from build123d import *

# Parameters (mm, degrees)
SKETCH1_W                = 13
SKETCH1_H                = 35
SKETCH1_R                = 3.175
BOSS_EXTRUDE1_DEPTH      = 101.6
CUT_EXTRUDE1_DEPTH       = 9
M4_CLEARANCE_HOLE1_D     = 4.3
M4_CLEARANCE_HOLE1_DEPTH = 5
M4_CLEARANCE_HOLE1_TIP   = 1.291850331
M4_CLEARANCE_HOLE2_D     = 4.3
M4_CLEARANCE_HOLE2_DEPTH = 5
M4_CLEARANCE_HOLE2_TIP   = 1.291850331
FILLET1_R                = 3


with BuildPart() as part:
    # Sketch1 → Boss-Extrude1 (new body)
    with BuildSketch(Plane.XY):
        with Locations((6.5, 17.5)):
            Rectangle(SKETCH1_W, SKETCH1_H)
        with Locations((6.5, 30)):
            Circle(SKETCH1_R, mode=Mode.SUBTRACT)
    extrude(amount=BOSS_EXTRUDE1_DEPTH)

    # Sketch2 → Cut-Extrude1 (cut, symmetric)
    with BuildSketch(Plane.XY.offset(75.25)):
        Polygon((0, 30), (0, 35), (13, 35), (13, 30), (13, 23.5), (0, 23.5), align=None)
    extrude(amount=CUT_EXTRUDE1_DEPTH, both=True, mode=Mode.SUBTRACT)

    # M4 Clearance Hole1
    with Locations(Plane(origin=(0, 0, 0), x_dir=(-1, 0, 0), z_dir=(0, 0, -1))):
        with Locations((-6.579246302, 18), (-6.579246302, 6)):
            Hole(M4_CLEARANCE_HOLE1_D / 2, depth=M4_CLEARANCE_HOLE1_DEPTH)
            with Locations((0, 0, -(M4_CLEARANCE_HOLE1_DEPTH + M4_CLEARANCE_HOLE1_TIP / 2))):  # 118° drill point
                Cone(0, M4_CLEARANCE_HOLE1_D / 2, M4_CLEARANCE_HOLE1_TIP, mode=Mode.SUBTRACT)

    # M4 Clearance Hole2
    with Locations(Plane.XY.offset(101.6)):
        with Locations((6.579246302, 18), (6.579246302, 6)):
            Hole(M4_CLEARANCE_HOLE2_D / 2, depth=M4_CLEARANCE_HOLE2_DEPTH)
            with Locations((0, 0, -(M4_CLEARANCE_HOLE2_DEPTH + M4_CLEARANCE_HOLE2_TIP / 2))):  # 118° drill point
                Cone(0, M4_CLEARANCE_HOLE2_D / 2, M4_CLEARANCE_HOLE2_TIP, mode=Mode.SUBTRACT)

    # Fillet1
    fillet1_edges = [part.edges().sort_by_distance(p)[0] for p in [
        (0, 35, 33.125),
        (13, 35, 33.125),
        (0, 35, 92.925),
        (13, 35, 92.925),
        (13, 0, 50.8),
        (0, 0, 50.8),
    ]]
    fillet(fillet1_edges, radius=FILLET1_R)


solid = part.part
Design review of the part built by this model. Coordinates are the model's own, in mm. A direction names the side the tool comes from. Round coordinates to 2 decimals unless told otherwise and drop trailing zeros. Loops run counter-clockwise (first coordinate to the right, second up) from the corner with the lowest first, then second, coordinate; pieces in that order, holes last. Notation, with made-up numbers: M -16.75,53.25 L 8.25,53.25 A36 cw 8.25,88.25 Z; hole C 41,-4 d6. An arc over 180 degrees is marked long. Answer as a JSON object with one key per item and string values.
Item 1: The part is to be moulded in two halves that separate along X. For faces 4 (the conical face through (6.223, 18.112, 6.067)), 5 (the cylindrical face through (0.86, 0.9, 51.51)), 6 (the cylindrical face through (12.1, 34.14, 33.59)), say which applies: pulls with the +X half, pulls with the -X half, needs draft (parallel to the pull), parting line crosses it, or undercut.
Answer sheet:
{"face 4": "undercut", "face 5": "pulls with the -X half", "face 6": "pulls with the +X half"}
Item 2: We need section C-C on x = 11.75. Give the boundary of the cut face in (y, z).
Answer sheet:
{"outline": "M 0.56,0 L 34.44,0 L 34.44,66.25 L 23.5,66.25 L 23.5,84.25 L 34.44,84.25 L 34.44,101.6 L 0.56,101.6 Z"}
Item 3: Wall thickness on L1, parallel to X at y = 18, z = 97.8; L2, parallel to Z at x = 11.25, y = 33.5; L3, parallel to X at y = 30, z = 37 (3 decimals): over which ranges is each line inside the solid? List them lowest first. Write a range as from..to.
Answer sheet:
{"L1": "x = 0..4.43, 8.73..13", "L2": "z = 0..66.25, 84.25..101.6", "L3": "x = 0..3.325, 9.675..13"}
Item 4: We need section A-A on y = 30. Give the boundary of the cut face in (x, z) (3 decimals), and give its area (3 significant figures).
Answer sheet:
{"outline": "M 0,0 L 3.325,0 L 3.325,66.25 L 0,66.25 Z; M 0,84.25 L 3.325,84.25 L 3.325,101.6 L 0,101.6 Z; M 9.675,0 L 13,0 L 13,66.25 L 9.675,66.25 Z; M 9.675,84.25 L 13,84.25 L 13,101.6 L 9.675,101.6 Z", "area": "556 mm^2"}
Item 5: Machinability: for faces 1 (the cylindrical face through (4.53, 6.65, 99.06)), 2 (the flat face through (7, 23.5, 75)), 3 (the cylindrical face through (6.11, 15.9, 2.54)), which of the approach directions +Z, -Z, +X, -X, +Y, -Y give a long, thin tool a straight path to every point of the face, cutting with its end or side? Answer none if there is none.
Answer sheet:
{"face 1": "+Z", "face 2": "+X, -X, +Y", "face 3": "-Z"}
Item 6: We need section B-B on z = 57. Give the boundary of the cut face in (x, y) (3 decimals), and give its area (3 significant figures).
Answer sheet:
{"outline": "M 0,3 A3 ccw 3,0 L 10,0 A3 ccw 13,3 L 13,32 A3 ccw 10,35 L 3,35 A3 ccw 0,32 Z; hole C 6.5,30 d6.35", "area": "416 mm^2"}
Item 7: Clearance check with flat-ended pins moving along their axes: P1, Ø5, axis at x = 6.5, y = 30, coming from the +Z side; P2, Ø4, axis at x = 6.58, y = 6, coming from the +Z side; P3, Ø3.5, axis at x = 6.58, y = 18, coming from the +Z side; P4, Ø5, axis at x = 5, z = 81.5, coming from the +Y side. State where each tip first meets the part, or that it passes through.
Answer sheet:
{"P1": "passes through", "P2": "stops at z = 96.51", "P3": "stops at z = 96.36", "P4": "stops at y = 23.5"}
